The model under review builds one solid part; all positions refer to its coordinate system, in mm. A direction names the side the tool comes from. Coordinates: 2 decimals unless noted, no trailing zeros. Loops run counter-clockwise (first coordinate to the right, second up) from the corner with the lowest first, then second, coordinate; pieces in that order, holes last. Notation, with made-up numbers: (-36.5, -33.75) - (-21.5, -33.75) arc R13 ccw to (-21.5, -25.75) - close; hole circle Ø4 at (80.5, 34). An arc over 180 degrees is marked (long way). Use a Markdown table: item, result. Add a question column.
1) Add section D-D, the plane z = 2.75. Give the boundary of the cut face in (x, y), and give its area (3 significant figures).
2) For faces 4 (the flat face through (23.91, -45, 12)), 5 (the flat face through (31, -14, 9)), 6 (the cylindrical face through (31.2, -28.6, 10.5)), 7 (the flat face through (13, 4, 5)), list the 3-axis set-ups (+Z, -Z, +X, -X, +Y, -Y) from which the entire face can be reached by the end or side of a thin tool; tool diameter is ignored.
3) To check wall thickness, follow L1, parallel to Y at x = 28.2, z = 7.6; L2, parallel to Y at x = -2.2, z = 6.65; L3, parallel to X at y = -27, z = 5.25. State the ranges of each line that lie inside material, in increasing order. Write a range as [from, to].
4) Add section B-B, the plane y = -43.75. Give the number of separate pieces and of enclosed holes in the cut face, and give its area (3 significant figures).
5) The part is to be moulded in two halves that separate along X. For faces 1 (the cylindrical face through (23.7, -28.6, 8.5)), 2 (the flat face through (48, -26, -5)), 3 (the flat face through (-20, -26, 5)), say which applies: pulls with the +X half, pulls with the -X half, needs draft (parallel to the pull), parting line crosses it, or undercut.
6) Add section A-A, the plane z = -7. Give the boundary of the cut face in (x, y), and give its area (3 significant figures).
7) Clearance check with flat-ended pins moving along their axes: pin 1 (4 mm diameter, centred on x = 11.5, z = 8, fed in from +Y); pin 2 (0.5 mm diameter, centred on y = -55.5, z = 6, fed in from -X); pin 3 (2 mm diameter, centred on x = 26.5, z = 12, fed in from +Y). State where each tip first meets the part, or that it passes through.
```python
from build123d import *

# Parameters (mm, degrees)
PAD007_DEPTH      = 46.5
SKETCH012_W       = 58
SKETCH012_H       = 2
PAD008_DEPTH      = 46.5
SKETCH013_W       = 2
SKETCH013_H       = 46.5
PAD009_DEPTH      = 62
SKETCH014_W       = 2
SKETCH014_H       = 46.5
PAD010_DEPTH      = 4
SKETCH015_W       = 66
SKETCH015_H       = 2
PAD011_DEPTH      = 7.25
SKETCH016_W       = 66
SKETCH016_H       = 2
PAD012_DEPTH      = 7.25
SKETCH017_W       = 66
SKETCH017_H       = 61
PAD013_DEPTH      = 9.8
SKETCH018_W       = 66
SKETCH018_H       = 61
PAD014_DEPTH      = 1.2
PAD015_DEPTH      = 5
SKETCH020_R       = 2.8
POCKET003_DEPTH   = 5
SKETCH021_R       = 1.5
POCKET004_DEPTH   = 8
SKETCH031_W       = 3.2
SKETCH031_H       = 7
POCKET010_DEPTH   = 5
FILLET_R          = 5
POCKET011_DEPTH   = 11
SKETCH034_W       = 33.6
SKETCH034_H       = 1.8
POCKET012_DEPTH   = 1.4
SKETCH035_W       = 70
SKETCH035_H       = 65
SKETCH035_W_2     = 66
SKETCH035_H_2     = 61
PAD019_DEPTH      = 9
PAD019_DEPTH_BACK = 0.1
FILLET001_R       = 1
FILLET002_R       = 0.99
SKETCH036_W       = 66.4
SKETCH036_H       = 61.4
POCKET013_DEPTH   = 9
SKETCH037_W       = 4.2
SKETCH037_H       = 8
POCKET014_DEPTH   = 5
SKETCH038_R       = 3
POCKET015_DEPTH   = 5
SKETCH039_R       = 1.6
POCKET016_DEPTH   = 5


with BuildPart() as part:
    # Sketch011 (on DatumPlane) → Pad007 (new body)
    with BuildSketch(Plane.XZ.offset(3.25)):
        with BuildLine():
            Line((-5, 11), (-16, 11))
            Line((-16, 11), (-16, 6))
            Line((-16, 6), (-15.726136, 6))
            ThreePointArc((-5.273864, 6), (-10.5, 10.75), (-15.726136, 6))
            Line((-5.273864, 6), (-5, 6))
            Line((-5, 6), (-5, 11))
        make_face()
    extrude(amount=PAD007_DEPTH)

    # Sketch012 (on DatumPlane) → Pad008 (join)
    with BuildSketch(Plane.XZ.offset(3.25)):
        with BuildLine():
            Line((42, 11), (31, 11))
            Line((31, 11), (31, 6))
            Line((31, 6), (31.273864, 6))
            ThreePointArc((41.726136, 6), (36.5, 10.75), (31.273864, 6))
            Line((41.726136, 6), (42, 6))
            Line((42, 6), (42, 11))
        make_face()
        with Locations((13, 12)):
            Rectangle(SKETCH012_W, SKETCH012_H)
    extrude(amount=PAD008_DEPTH)

    # Sketch013 (on Face17 of Pad008) → Pad009 (join)
    with BuildSketch(Plane(origin=(42, -3.25, 0), x_dir=(0, 0, 1), z_dir=(1, 0, 0))):
        with Locations((12, 23.25)):
            Rectangle(SKETCH013_W, SKETCH013_H)
    extrude(amount=-PAD009_DEPTH)

    # Sketch014 (on Face17 of Pad009) → Pad010 (join)
    with BuildSketch(Plane(origin=(42, -3.25, 0), x_dir=(0, 0, 1), z_dir=(1, 0, 0))):
        with Locations((12, 23.25)):
            Rectangle(SKETCH014_W, SKETCH014_H)
    extrude(amount=PAD010_DEPTH)

    # Sketch015 (on Face10 of Pad010) → Pad011 (join)
    with BuildSketch(Plane(origin=(0, -3.25, 0), x_dir=(1, 0, 0), z_dir=(0, 1, 0))):
        with Locations((13, -12)):
            Rectangle(SKETCH015_W, SKETCH015_H)
    extrude(amount=PAD011_DEPTH)

    # Sketch016 (on Face12 of Pad011) → Pad012 (join)
    with BuildSketch(Plane.XZ.offset(49.75)):
        with Locations((13, 12)):
            Rectangle(SKETCH016_W, SKETCH016_H)
    extrude(amount=PAD012_DEPTH)

    # Sketch017 (on Face14 of Pad012) → Pad013 (join)
    with BuildSketch(Plane(origin=(0, -3.25, 11), x_dir=(1, 0, 0), z_dir=(0, 0, -1))):
        with Locations((13, 23.25)):
            Rectangle(SKETCH017_W, SKETCH017_H)
        Polygon((42.2, -4.45), (-16.2, -4.45), (-16.2, 50.95), (22.8, 50.95), (22.8, 52.25), (31.2, 52.25), (31.2, 50.95), (42.2, 50.95), align=None, mode=Mode.SUBTRACT)
    extrude(amount=PAD013_DEPTH)

    # Sketch018 (on Face18 of Pad013) → Pad014 (join)
    with BuildSketch(Plane(origin=(0, -3.25, 1.2), x_dir=(1, 0, 0), z_dir=(0, 0, -1))):
        with Locations((13, 23.25)):
            Rectangle(SKETCH018_W, SKETCH018_H)
        Polygon((-2.2, 52.95), (31.2, 52.95), (31.2, 50.95), (42.2, 50.95), (42.2, -4.45), (-16.2, -4.45), (-16.2, 50.95), (-2.2, 50.95), align=None, mode=Mode.SUBTRACT)
    extrude(amount=PAD014_DEPTH)

    # Sketch019 (on Face13 of Pad014) → Pad015 (join)
    with BuildSketch(Plane(origin=(0, -3.25, 11), x_dir=(1, 0, 0), z_dir=(0, 0, -1))):
        with BuildLine():
            ThreePointArc((-5, 36.977217), (2.3, 40.5), (-5, 44.022783))
            Line((-5, 44.022783), (-5, 36.977217))
        make_face()
        with BuildLine():
            ThreePointArc((-5, 6.477217), (2.3, 10), (-5, 13.522783))
            Line((-5, 13.522783), (-5, 6.477217))
        make_face()
        with BuildLine():
            ThreePointArc((31, 28.772783), (23.7, 25.25), (31, 21.727217))
            Line((31, 28.772783), (31, 21.727217))
        make_face()
    extrude(amount=PAD015_DEPTH)

    # Sketch020 (on Face67 of Pad015) → Pocket003 (cut)
    with BuildSketch(Plane(origin=(0, -3.25, 13), x_dir=(-1, 0, 0), z_dir=(0, 0, 1))):
        with Locations((2.2, 40.5)):
            Circle(SKETCH020_R)
        with Locations((2.2, 10)):
            Circle(SKETCH020_R)
        with Locations((-28.2, 25.25)):
            Circle(SKETCH020_R)
    extrude(amount=-POCKET003_DEPTH, mode=Mode.SUBTRACT)

    # Sketch021 (on Face67 of Pocket003) → Pocket004 (cut)
    with BuildSketch(Plane(origin=(0, -3.25, 13), x_dir=(-1, 0, 0), z_dir=(0, 0, 1))):
        with Locations((-28.2, 25.25)):
            Circle(SKETCH021_R)
        with Locations((2.2, 10)):
            Circle(SKETCH021_R)
        with Locations((2.2, 40.5)):
            Circle(SKETCH021_R)
    extrude(amount=-POCKET004_DEPTH, mode=Mode.SUBTRACT)

    # Sketch031 (on Face14 of Pocket004) → Pocket010 (cut)
    with BuildSketch(Plane(origin=(0, -3.25, 11), x_dir=(1, 0, 0), z_dir=(0, 0, -1))):
        with Locations((26.01, 42.05)):
            Rectangle(SKETCH031_W, SKETCH031_H)
    extrude(amount=-POCKET010_DEPTH, mode=Mode.SUBTRACT)

    # Fillet
    fillet_edges = [part.edges().sort_by_distance(p)[0] for p in [
        (-20, -26.5, 13),
        (-20, -53.375, 13),
        (13, -57, 13),
        (46, -53.375, 13),
        (46, -26.5, 13),
        (46, 0.375, 13),
        (13, 4, 13),
        (-20, 0.375, 13),
    ]]
    fillet(fillet_edges, radius=FILLET_R)

    # Sketch033 (on Face30 of Fillet) → Pocket011 (cut)
    with BuildSketch(Plane(origin=(0, -3.25, 11), x_dir=(1, 0, 0), z_dir=(0, 0, -1))):
        Polygon((22.6, 51.15), (-16.4, 51.15), (-16.4, -4.65), (42.4, -4.65), (42.4, 51.15), (31.4, 51.15), (31.4, 52.45), (22.6, 52.45), align=None)
        Polygon((-16.2, 50.95), (-16.2, -4.45), (42.2, -4.45), (42.2, 50.95), (31.2, 50.95), (31.2, 52.25), (22.8, 52.25), (22.8, 50.95), align=None, mode=Mode.SUBTRACT)
    extrude(amount=POCKET011_DEPTH, mode=Mode.SUBTRACT)

    # Sketch034 (on Face44 of Pocket011) → Pocket012 (cut)
    with BuildSketch(Plane(origin=(0, -3.25, 0), x_dir=(1, 0, 0), z_dir=(0, 0, -1))):
        with Locations((14.6, 52.05)):
            Rectangle(SKETCH034_W, SKETCH034_H)
    extrude(amount=-POCKET012_DEPTH, mode=Mode.SUBTRACT)

    # Sketch035 (on Face44 of Pocket012) → Pad019 (join, two sides)
    with BuildSketch(Plane(origin=(0, -3.25, 0), x_dir=(1, 0, 0), z_dir=(0, 0, -1))) as pad019_sk:
        with Locations((13, 23.25)):
            Rectangle(SKETCH035_W, SKETCH035_H)
        with Locations((13, 23.25)):
            Rectangle(SKETCH035_W_2, SKETCH035_H_2, mode=Mode.SUBTRACT)
    extrude(amount=PAD019_DEPTH)
    extrude(pad019_sk.sketch, amount=-PAD019_DEPTH_BACK)

    # Fillet001
    fillet001_edges = [part.edges().sort_by_distance(p)[0] for p in [
        (46, -26.5, 0.1),
        (13, 4, 0.1),
        (-20, -26.5, 0.1),
        (13, -57, 0.1),
    ]]
    fillet(fillet001_edges, radius=FILLET001_R)

    # Fillet002
    fillet002_edges = [part.edges().sort_by_distance(p)[0] for p in [
        (13, 6, 0.1),
        (-22, -26.5, 0.1),
        (48, -26.5, 0.1),
        (13, -59, 0.1),
    ]]
    fillet(fillet002_edges, radius=FILLET002_R)

    # Sketch036 (on Face18 of Fillet002) → Pocket013 (cut)
    with BuildSketch(Plane(origin=(0, -3.25, -9), x_dir=(1, 0, 0), z_dir=(0, 0, -1))):
        with Locations((13, 23.25)):
            Rectangle(SKETCH036_W, SKETCH036_H)
    extrude(amount=-POCKET013_DEPTH, mode=Mode.SUBTRACT)

    # Sketch037 (on Face58 of Pocket013) → Pocket014 (cut)
    with BuildSketch(Plane(origin=(0, -3.25, 11), x_dir=(1, 0, 0), z_dir=(0, 0, -1))):
        with Locations((26.01, 42.05)):
            Rectangle(SKETCH037_W, SKETCH037_H)
    extrude(amount=-POCKET014_DEPTH, mode=Mode.SUBTRACT)

    # Sketch038 (on Face37 of Pocket014) → Pocket015 (cut)
    with BuildSketch(Plane(origin=(0, -3.25, 13), x_dir=(-1, 0, 0), z_dir=(0, 0, 1))):
        with Locations((2.2, 40.5)):
            Circle(SKETCH038_R)
        with Locations((-28.2, 25.25)):
            Circle(SKETCH038_R)
        with Locations((2.2, 10)):
            Circle(SKETCH038_R)
    extrude(amount=-POCKET015_DEPTH, mode=Mode.SUBTRACT)

    # Sketch039 (on Face66 of Pocket015) → Pocket016 (cut)
    with BuildSketch(Plane(origin=(0, -3.25, 8), x_dir=(-1, 0, 0), z_dir=(0, 0, 1))):
        with Locations((2.2, 40.5)):
            Circle(SKETCH039_R)
        with Locations((-28.2, 25.25)):
            Circle(SKETCH039_R)
        with Locations((2.2, 10)):
            Circle(SKETCH039_R)
    extrude(amount=-POCKET016_DEPTH, mode=Mode.SUBTRACT)


solid = part.part
```
From the geometry:
| question | item | result |
|---|---|---|
| 1 | outline | (-20, -57) - (46, -57) - (46, 4) - (-20, 4) - close; hole (-16.4, -54.4) - (22.6, -54.4) - (22.6, -55.7) - (31.4, -55.7) - (31.4, -54.4) - (42.4, -54.4) - (42.4, 1.4) - (-16.4, 1.4) - close |
| 1 | area | 734 mm^2 |
| 2 | face 4 | +Z, -Z |
| 2 | face 5 | -Z |
| 2 | face 6 | +Z |
| 2 | face 7 | +Z, +X, -X, +Y |
| 3 | L1 | y = [-57, -55.7], [-33, -30.1], [-26.9, -24], [1.4, 4] |
| 3 | L2 | y = [-57, -54.4], [-48.25, -45.35], [-42.15, -39.25], [-17.75, -14.85], [-11.65, -8.75], [1.4, 4] |
| 3 | L3 | x = [-20, -16.4], [42.4, 46] |
| 4 | separate pieces | 3 |
| 4 | enclosed holes | 0 |
| 4 | area | 259 mm^2 |
| 5 | face 1 | undercut |
| 5 | face 2 | pulls with the +X half |
| 5 | face 3 | pulls with the -X half |
| 6 | outline | (-22, -59) - (48, -59) - (48, 6) - (-22, 6) - close; hole (-20.2, -57.2) - (46.2, -57.2) - (46.2, 4.2) - (-20.2, 4.2) - close |
| 6 | area | 473 mm^2 |
| 7 | pin 1 | stops at y = 4 |
| 7 | pin 2 | stops at x = -20 |
| 7 | pin 3 | stops at y = 3 |
